from build123d import *

# Parameters (mm, degrees)
Y_KSEKLIK_EKSTR_ZYON1_DEPTH = 20
IZIM2_R                     = 6
KES_EKSTR_ZYON1_DEPTH       = 20
IZIM3_R                     = 3
KES_EKSTR_ZYON2_DEPTH       = 40


with BuildPart() as part:
    # Çizim1 → Yükseklik-Ekstrüzyon1 (new body)
    with BuildSketch(Plane.XY):
        Polygon((-22.5, 14.5), (22.5, 14.5), (22.5, -14.5), (-22.5, -14.5), (-22.5, -10.5), (7.5, -10.5), (7.5, 10.5), (-22.5, 10.5), align=None)
    extrude(amount=Y_KSEKLIK_EKSTR_ZYON1_DEPTH)

    # Çizim2 → Kes-Ekstrüzyon1 (cut)
    with BuildSketch(Plane(origin=(22.5, 0, 0), x_dir=(0, 0, -1), z_dir=(1, 0, 0))):
        with Locations((-10, 0)):
            Circle(IZIM2_R)
    extrude(amount=-KES_EKSTR_ZYON1_DEPTH, mode=Mode.SUBTRACT)

    # Çizim3 → Kes-Ekstrüzyon2 (cut)
    with BuildSketch(Plane.XZ.offset(14.5)):
        with Locations((-16.5, 10)):
            Circle(IZIM3_R)
    extrude(amount=-KES_EKSTR_ZYON2_DEPTH, mode=Mode.SUBTRACT)


solid = part.part
The listing builds one solid part. Answer for the finished solid, in the listing's coordinates (mm). A direction names the side the tool comes from. Round coordinates to 2 decimals unless told otherwise and drop trailing zeros. Write each loop counter-clockwise with the first axis right and the second up, starting at its lowest first coordinate (ties: lowest second). Pieces come first, ordered by that corner, then holes. Notation, with made-up numbers: M 54,57 L 96,57 A36 ccw 96,96 Z; hole C 4,24 d9. An arc over 180 degrees is marked long. Write each question's results on one line, items separated by ' | '. Start each with the question number.
Item 1: For faces 1 (the face through (-7, 10.5, 10)), 2 (the face through (-22.5, -13, 10)), determine the directions among +Z, -Z, +X, -X, +Y, -Y from which every point of the face is accessible in a straight line to the end or side of a thin tool.
Item 2: For a pull along X with two mould halves and no side action, classify faces 3 (the face through (-19.5, -12.5, 10.1)), 4 (the face through (10, 0, 20)), 5 (the face through (-19.5, 12.5, 10.1)), 6 (the face through (22.5, -6.2, 9.9)) as pulls with the +X half, pulls with the -X half, needs draft (parallel to the pull), parting line crosses it, or undercut.
Item 3: A cutting plane is placed at C-C on y = 0. Write down the section's boundary in (x, z).
Item 4: A cutting plane is placed at D-D on x = -16.5. Write down the section's boundary in (y, z), and give its area (3 significant figures).
Item 5: A cutting plane is placed at B-B on x = -7.5. Write down the section's boundary in (y, z), and give its area (3 significant figures).
Item 6: Straight lines are drawn through the part: L1, parallel to Y at x = -20, z = 5.25; L2, parallel to Y at x = 16.5, z = 10; L3, parallel to Z at x = -16.5, y = 13.5. For each, find the intervals that lie inside material, in ascending order. Write a range as [from, to].
Item 7: A cutting plane is placed at A-A on z = 10. Write down the section's boundary in (x, y).
Item 8: A flat-ended cylindrical pin translates along its axis: pin 1 Ø2 at (y, z) = (-8.5, 9) entering from -X. Find the tip coordinate at first contact, or state that the pin passes through.
Check sheet entries:
1) face 1: +Z, -Z, -X | face 2: +Z, -Z, -X, +Y, -Y
2) face 3: undercut | face 4: needs draft | face 5: undercut | face 6: pulls with the +X half
3) outline: M 7.5,0 L 22.5,0 L 22.5,4 L 7.5,4 Z; M 7.5,16 L 22.5,16 L 22.5,20 L 7.5,20 Z
4) outline: M -14.5,0 L -10.5,0 L -10.5,7 L -14.5,7 Z; M -14.5,13 L -10.5,13 L -10.5,20 L -14.5,20 Z; M 10.5,0 L 14.5,0 L 14.5,7 L 10.5,7 Z; M 10.5,13 L 14.5,13 L 14.5,20 L 10.5,20 Z | area: 112 mm²
5) outline: M -14.5,0 L -10.5,0 L -10.5,20 L -14.5,20 Z; M 10.5,0 L 14.5,0 L 14.5,20 L 10.5,20 Z | area: 160 mm²
6) L1: [-14.5, -10.5], [10.5, 14.5] | L2: [-14.5, -6], [6, 14.5] | L3: [0, 7], [13, 20]
7) outline: M -22.5,-14.5 L -19.5,-14.5 L -19.5,-10.5 L -22.5,-10.5 Z; M -22.5,10.5 L -19.5,10.5 L -19.5,14.5 L -22.5,14.5 Z; M -13.5,-14.5 L 22.5,-14.5 L 22.5,-6 L 7.5,-6 L 7.5,-10.5 L -13.5,-10.5 Z; M -13.5,10.5 L 7.5,10.5 L 7.5,6 L 22.5,6 L 22.5,14.5 L -13.5,14.5 Z
8) pin 1: x = 7.5
